from build123d import *

# Parameters (mm, degrees)
SKETCH1_R           = 12.7
BOSS_EXTRUDE1_DEPTH = 25.4
SKETCH2_R           = 3.175
BOSS_EXTRUDE2_DEPTH = 25.4
SKETCH3_W           = 6.35
SKETCH3_H           = 6.35
BOSS_EXTRUDE3_DEPTH = 20.32
SKETCH4_R           = 1.5875
CUT_EXTRUDE1_DEPTH  = 55.716959208


with BuildPart() as part:
    # Sketch1 → Boss-Extrude1 (new, symmetric)
    with BuildSketch(Plane.XY):
        Circle(SKETCH1_R)
    extrude(amount=BOSS_EXTRUDE1_DEPTH, both=True)

    # Sketch2 → Boss-Extrude2 (add)
    with BuildSketch(Plane.XY.offset(25.4)):
        Circle(SKETCH2_R)
    extrude(amount=BOSS_EXTRUDE2_DEPTH)

    # Sketch3 → Boss-Extrude3 (add)
    with BuildSketch(Plane(origin=(0, 0, -25.4), x_dir=(-1, 0, 0), z_dir=(0, 0, -1))):
        Rectangle(SKETCH3_W, SKETCH3_H)
    extrude(amount=BOSS_EXTRUDE3_DEPTH)

    # Sketch4 → Cut-Extrude1 (cut, through all)
    with BuildSketch(Plane(origin=(0, 3.175, 0), x_dir=(1, 0, 0), z_dir=(0, 1, 0))):
        with Locations(Location((0, 41.91, 0), (0, 0, 270))):
            Circle(SKETCH4_R)
    extrude(amount=-CUT_EXTRUDE1_DEPTH, mode=Mode.SUBTRACT)


solid = part.part
Check sheet for the modelled part. Datum: model origin and axes. Units: mm. A direction names the side the tool comes from. Give positions to 0.01 mm unless a question says otherwise; leave off trailing zeros. Order: outer loops, then holes, each group sorted by start corner. A loop starts at its lowest first (then second) coordinate and runs counter-clockwise, first axis right, second up. Notation, with made-up numbers: M 13.25,38.25 L 69.25,38.25 A19 cw 69.25,46.25 Z; hole C 69,-23.5 d7. An arc over 180 degrees is marked long. Answer as CSV lines item,"result". Start each with the question number.
Item 1: Mould release check, pull along X, two halves, no side actions. Record for faces 1 (the face through (-0.69, -3.1, 37.92)), 2 (the face through (0.07, 0.044, -43.496)), 3 (the face through (5, 0, -25.4)): +X half, -X half, draft (parallel to the pull), parting line (faces both ways), or undercut.
Item 2: Cross-section at C-C on z = -5.5. Enter the section's corners in (x, y).
Item 3: Cross-section at A-A on y = 0. Enter the section's corners in (x, z) (1 decimal).
Item 4: Cross-section at D-D on x = 4.75. Enter the section's corners in (y, z), plus the area to 3 significant figures.
Item 5: Thickness scan on line 1 (Z direction, x = 5.75, y = -5.5); line 2 (X direction, y = -0.5, z = -41.91) (1 decimal); line 3 (Y direction, x = 0, z = 26) (3 decimals). Record the ranges inside material, lowest first. Write a range as [from, to].
Item 6: Cross-section at B-B on z = -41.91. Enter the section's corners in (x, y) (1 decimal).
Item 7: Tool access check on faces 4 (the face through (-3.175, 0, -35)), 5 (the face through (0, -3.175, -35)), 6 (the face through (3, -3, 25.4)), 7 (the face through (0, 3.175, -35)), 8 (the face through (3.175, 0, -35)). Record the directions out of +Z, -Z, +X, -X, +Y, -Y that give a thin tool (end or side, any length) a straight path to the whole face; none if there is none.
Item 8: Gauge pin test, flat ends, axial feed: P1, Ø5, axis at y = 1.5, z = -39, coming from the -X side (3 decimals); P2, Ø4, axis at x = 0, z = -41.91, coming from the -Y side (3 decimals); P3, Ø1.9, axis at y = 0.5, z = -32.5, coming from the +X side (3 decimals). Record the tip position at first contact, or that the pin passes through.
Established:
1,face 1,"parting line"
1,face 2,"undercut"
1,face 3,"draft"
2,outline,"C 0,0 d25.4"
3,outline,"M -12.7,-25.4 L -3.2,-25.4 L -3.2,-45.7 L 3.2,-45.7 L 3.2,-25.4 L 12.7,-25.4 L 12.7,25.4 L 3.2,25.4 L 3.2,50.8 L -3.2,50.8 L -3.2,25.4 L -12.7,25.4 Z; hole C 0,-41.9 d3.2"
4,outline,"M -11.78,-25.4 L 11.78,-25.4 L 11.78,25.4 L -11.78,25.4 Z"
4,area,"1,200 mm^2"
5,line 1,"z = [-25.4, 25.4]"
5,line 2,"x = [-3.2, -1.6], [1.6, 3.2]"
5,line 3,"y = [-3.175, 3.175]"
6,outline,"M -3.2,-3.2 L -1.6,-3.2 L -1.6,3.2 L -3.2,3.2 Z; M 1.6,-3.2 L 3.2,-3.2 L 3.2,3.2 L 1.6,3.2 Z"
7,face 4,"-Z, -X, +Y, -Y"
7,face 5,"-Z, +X, -X, -Y"
7,face 6,"+Z"
7,face 7,"-Z, +X, -X, +Y"
7,face 8,"-Z, +X, +Y, -Y"
8,P1,"stops at x = -3.175"
8,P2,"stops at y = -3.175"
8,P3,"stops at x = 3.175"
